The model under review builds one solid part; all positions refer to its coordinate system, in mm. A direction names the side the tool comes from. Coordinates: 2 decimals unless noted, no trailing zeros. Order: outer loops, then holes, each group sorted by start corner. A loop starts at its lowest first (then second) coordinate and runs counter-clockwise, first axis right, second up.
```python
from build123d import *

# Parameters (mm, degrees)
F0_W     = 30
F0_H     = 30
F1_DEPTH = 2
F2_R     = 12.5
F3_DEPTH = 2
F5_DEPTH = 2


with BuildPart() as f1:
    # F0 (on Top) → F1 (new body)
    with BuildSketch(Plane.XY):
        Rectangle(F0_W, F0_H)
    extrude(amount=F1_DEPTH)

    # F2 (on face) → F3 (join)
    with BuildSketch(Plane.XY.offset(2)):
        Circle(F2_R)
    extrude(amount=F3_DEPTH)

    # F4 (on face) → F5 (join)
    with BuildSketch(Plane.XY.offset(4)):
        Polygon((0, 11.547005), (-10, 5.773503), (-10, -5.773503), (0, -11.547005), (10, -5.773503), (10, 5.773503), align=None)
    extrude(amount=F5_DEPTH)


solid = f1.part
```
(1) We need section A-A, the plane z = 5.45. Write out the cut boundary in (x, y).
A:
outline: (-10, -5.77) - (0, -11.55) - (10, -5.77) - (10, 5.77) - (0, 11.55) - (-10, 5.77) - close
(2) For pin 1 Ø1.5 at (y, z) = (2, 5) entering from -X; pin 2 Ø2 at (x, y) = (12, 3.5) entering from +Z; pin 3 Ø1.6 at (y, z) = (-1, 5) entering from +X, all flat-tipped, find the tip position at first contact; note any pin that passes through.
A:
pin 1: stops at x = -10
pin 2: stops at z = 4
pin 3: stops at x = 10
(3) Machinability: for faces 1 (the face through (10, 0, 5)), 2 (the face through (-4.93, 8.7, 4.99)), 3 (the face through (5.07, 8.62, 4.99)), 4 (the face through (5, 9, 4)), which of the approach directions +Z, -Z, +X, -X, +Y, -Y give a long, thin tool a straight path to every point of the face, cutting with its end or side? Answer none if there is none.
A:
face 1: +Z, +X, +Y, -Y
face 2: +Z, -X, +Y
face 3: +Z, +X, +Y
face 4: +Z
(4) We need section D-D, the plane z = 2.95. Write out the cut boundary in (x, y), and give its area (3 significant figures).
A:
outline: circle Ø25 at (0, 0)
area: 491 mm2
(5) We need section B-B, the plane y = 0. Write out the cut boundary in (x, z).
A:
outline: (-15, 0) - (15, 0) - (15, 2) - (12.5, 2) - (12.5, 4) - (10, 4) - (10, 6) - (-10, 6) - (-10, 4) - (-12.5, 4) - (-12.5, 2) - (-15, 2) - close
(6) Wall thickness on probe 1 along X at (y, z) = (-3.5, 4.1); probe 2 along Z at (x, y) = (10.75, 13): over which ranges is each line inside the solid? List them lowest first.
A:
probe 1: x = -10 to 10
probe 2: z = 0 to 2
(7) We need section C-C, the plane x = 5.5. Write out the cut boundary in (y, z).
A:
outline: (-15, 0) - (15, 0) - (15, 2) - (11.22, 2) - (11.22, 4) - (8.37, 4) - (8.37, 6) - (-8.37, 6) - (-8.37, 4) - (-11.22, 4) - (-11.22, 2) - (-15, 2) - close
